Could you check a few things on this drawing? It's one solid part, dimensions in mm from its lowest x, y, z. Round coordinates to 2 decimals unless told otherwise and drop trailing zeros. Answer as a JSON object with one key per item and string values.
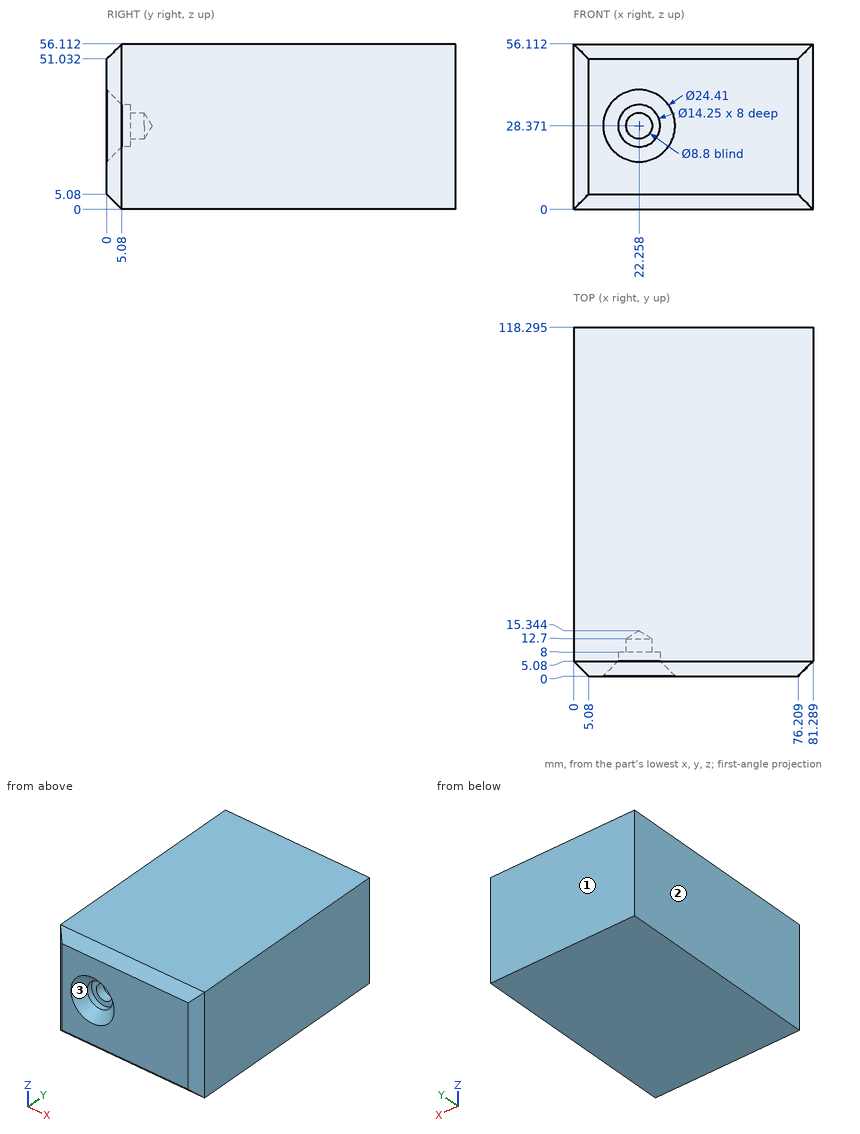
Item 1: If we mould it in two halves opening along X, with no side actions, what happens to the marked faces 1, 2 and 3? For each: pulls with the +X half, pulls with the -X half, needs draft (parallel to the pull), parting line crosses it, or undercut.
Resolved:
{"face 1": "needs draft", "face 2": "pulls with the -X half", "face 3": "undercut"}
Item 2: I'm going to push flat-ended pins straight in: pin 1 Ø18.5 at (x, z) = (22.26, 28.37) entering from -Y; pin 2 Ø4.5 at (x, z) = (25.5, 28) entering from -Y. Where does each tip first touch, or does it pass through?
Resolved:
{"pin 1": "y = 2.95", "pin 2": "y = 8"}
Item 3: Please list where these lines run through material, in increasing order: probe 1 along Y at (x, z) = (29, 27.5) (1 decimal); probe 2 along Y at (x, z) = (29, 4) (1 decimal). Write a range as from..to.
Resolved:
{"probe 1": "8..118.3", "probe 2": "1.1..118.3"}
